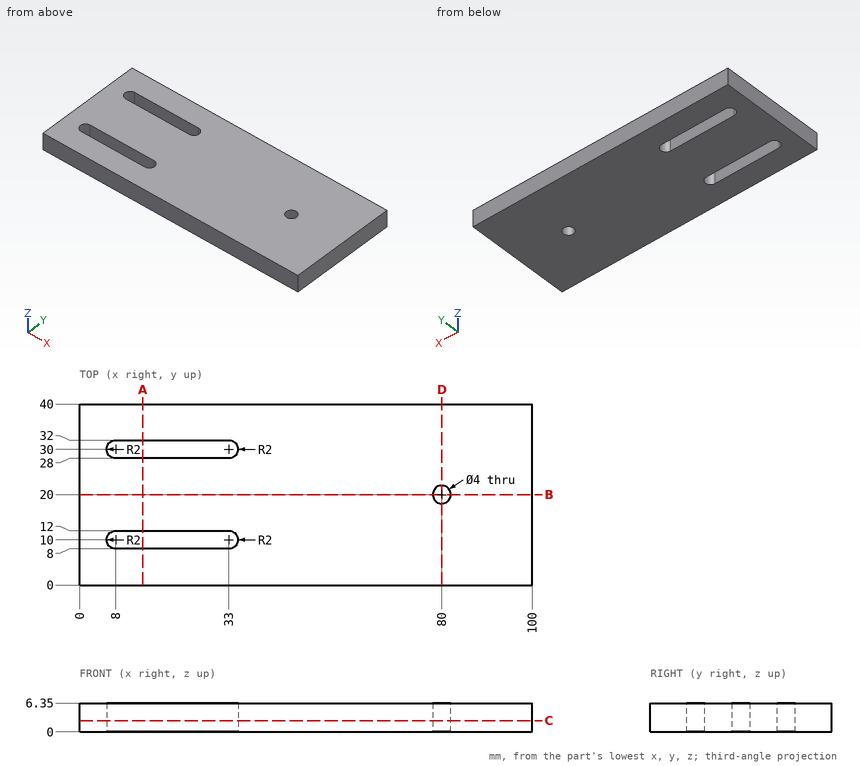
Design review of the part shown in the three views and the two pictorial views. Dimensions are in mm from the part's minimum x, y and z. Give positions to 0.01 mm unless a question says otherwise; leave off trailing zeros. Loops run counter-clockwise (first coordinate to the right, second up) from the corner with the lowest first, then second, coordinate; pieces in that order, holes last. Notation, with made-up numbers: (80.5, 71.25) -> (107.5, 71.25) arc R27 ccw to (107.5, 91.25) -> close; hole circle Ø11 at (15.25, 15). An arc over 180 degrees is marked (long way). Write each question's results on one line, items separated by ' | '.
1) Take a section at A-A, the plane x = 14. Give the boundary of the cut face in (y, z).
Conclusion:
outline: (0, 0) -> (8, 0) -> (8, 6.35) -> (0, 6.35) -> close; (12, 0) -> (28, 0) -> (28, 6.35) -> (12, 6.35) -> close; (32, 0) -> (40, 0) -> (40, 6.35) -> (32, 6.35) -> close
2) Take a section at B-B, the plane y = 20. Give the boundary of the cut face in (x, z).
Conclusion:
outline: (0, 0) -> (78, 0) -> (78, 6.35) -> (0, 6.35) -> close; (82, 0) -> (100, 0) -> (100, 6.35) -> (82, 6.35) -> close
3) Take a section at D-D, the plane x = 80. Give the boundary of the cut face in (y, z).
Conclusion:
outline: (0, 0) -> (18, 0) -> (18, 6.35) -> (0, 6.35) -> close; (22, 0) -> (40, 0) -> (40, 6.35) -> (22, 6.35) -> close
4) Take a section at C-C, the plane z = 2.5. Give the boundary of the cut face in (x, y).
Conclusion:
outline: (0, 0) -> (100, 0) -> (100, 40) -> (0, 40) -> close; hole (8, 8) -> (33, 8) arc R2 ccw to (33, 12) -> (8, 12) arc R2 ccw to start; hole (8, 28) -> (33, 28) arc R2 ccw to (33, 32) -> (8, 32) arc R2 ccw to start; hole circle Ø4 at (80, 20)
5) For line 1 along Y through (x, z) = (12.5, 2.25); line 2 along Y through (x, z) = (80, 3.5); line 3 along X through (y, z) = (29.5, 3.25), list the stretches that pass through material, from the lowest coordinate up. Write a range as from..to.
Conclusion:
line 1: y = 0..8, 12..28, 32..40 | line 2: y = 0..18, 22..40 | line 3: x = 0..6.06, 34.94..100
